from build123d import *

# Parameters (mm, degrees)
F1_DEPTH  = 12.7
F1_FACE_R = 30.3566666554
F2_DEPTH  = 12.7


with BuildPart() as f1:
    # F0 (on Front) → F1 (new body)
    with BuildSketch(Plane.XZ):
        with BuildLine():
            ThreePointArc((-9.3004843115, 36.7589222648), (-23.2923661717, -29.9196098341), (37.9172437619, 0))
            ThreePointArc((37.9172437619, 0), (29.338119554, 24.020660181), (7.4829580234, 37.1715309574))
            Line((7.4829580234, 37.1715309574), (0, 30.3566666554))
            Line((0, 30.3566666554), (-9.3004843115, 36.7589222648))
        make_face()
        with BuildLine():
            ThreePointArc((30.3566666554, 0), (-21.4654048463, -21.4654048463), (0, 30.3566666554))
            ThreePointArc((0, 30.3566666554), (21.4654048463, 21.4654048463), (30.3566666554, 0))
        make_face(mode=Mode.SUBTRACT)
        with BuildLine():
            Line((0, 30.3566666554), (7.4829580234, 37.1715309574))
            ThreePointArc((7.4829580234, 37.1715309574), (-0.9318862244, 37.9057906205), (-9.3004843115, 36.7589222648))
            Line((-9.3004843115, 36.7589222648), (0, 30.3566666554))
        make_face()
        with BuildLine():
            ThreePointArc((-9.3004843115, 36.7589222648), (-0.9318862244, 37.9057906205), (7.4829580234, 37.1715309574))
            Line((7.4829580234, 37.1715309574), (20.2197378858, 48.7711451921))
            ThreePointArc((20.2197378858, 48.7711451921), (11.7747091364, 46.8406854256), (3.6217325155, 49.7688516961))
            ThreePointArc((3.6217325155, 49.7688516961), (-6.3831384952, 42.0012170686), (-18.9701891405, 43.4153414263))
            Line((-18.9701891405, 43.4153414263), (-9.3004843115, 36.7589222648))
        make_face()
        with BuildLine():
            ThreePointArc((3.6217325155, 49.7688516961), (11.7747091364, 46.8406854256), (20.2197378858, 48.7711451921))
            Line((20.2197378858, 48.7711451921), (25.3996234387, 53.4885600209))
            Line((25.3996234387, 53.4885600209), (0, 70.9731206298))
            ThreePointArc((0, 70.9731206298), (4.3420940931, 65.2280612526), (5.8836441513, 58.193637909))
            ThreePointArc((5.8836441513, 58.193637909), (5.3083274131, 53.8320651714), (3.6217325155, 49.7688516961))
        make_face()
        with BuildLine():
            Line((25.3996234387, 53.4885600209), (20.2197378858, 48.7711451921))
            ThreePointArc((20.2197378858, 48.7711451921), (23.0811869033, 50.8317293109), (25.3996234387, 53.4885600209))
        make_face()
        with BuildLine():
            ThreePointArc((-21.873843285, 45.4141551882), (-20.4745226574, 44.3384727889), (-18.9701891405, 43.4153414263))
            Line((-18.9701891405, 43.4153414263), (-21.873843285, 45.4141551882))
        make_face()
        with BuildLine():
            Line((-21.873843285, 45.4141551882), (-18.9701891405, 43.4153414263))
            ThreePointArc((-18.9701891405, 43.4153414263), (-6.3831384952, 42.0012170686), (3.6217325155, 49.7688516961))
            ThreePointArc((3.6217325155, 49.7688516961), (-2.498029855, 59.6350178914), (0, 70.9731206298))
            Line((0, 70.9731206298), (-21.873843285, 45.4141551882))
        make_face()
        with BuildLine():
            Line((0, 70.9731206298), (25.3996234387, 53.4885600209))
            ThreePointArc((25.3996234387, 53.4885600209), (27.4225414081, 57.653295881), (28.1177455183, 62.2308403254))
            ThreePointArc((28.1177455183, 62.2308403254), (17.2773561637, 76.9535700141), (0, 70.9731206298))
        make_face()
        with BuildLine():
            ThreePointArc((0, 70.9731206298), (-2.498029855, 59.6350178914), (3.6217325155, 49.7688516961))
            ThreePointArc((3.6217325155, 49.7688516961), (5.3083274131, 53.8320651714), (5.8836441513, 58.193637909))
            ThreePointArc((5.8836441513, 58.193637909), (4.3420940931, 65.2280612526), (0, 70.9731206298))
        make_face()
        with BuildLine():
            ThreePointArc((0, 70.9731206298), (-23.7164043633, 69.1305595515), (-21.873843285, 45.4141551882))
            Line((-21.873843285, 45.4141551882), (0, 70.9731206298))
        make_face()
    extrude(amount=-F1_DEPTH)

    # F0 (on Front) + F1_face (on face) → F2 (join)
    with BuildSketch(Plane.XZ):
        with BuildLine():
            ThreePointArc((-9.3004843115, 36.7589222648), (-23.2923661717, -29.9196098341), (37.9172437619, 0))
            ThreePointArc((37.9172437619, 0), (29.338119554, 24.020660181), (7.4829580234, 37.1715309574))
            Line((7.4829580234, 37.1715309574), (0, 30.3566666554))
            Line((0, 30.3566666554), (-9.3004843115, 36.7589222648))
        make_face()
        with BuildLine():
            ThreePointArc((30.3566666554, 0), (-21.4654048463, -21.4654048463), (0, 30.3566666554))
            ThreePointArc((0, 30.3566666554), (21.4654048463, 21.4654048463), (30.3566666554, 0))
        make_face(mode=Mode.SUBTRACT)
        with BuildLine():
            Line((0, 30.3566666554), (7.4829580234, 37.1715309574))
            ThreePointArc((7.4829580234, 37.1715309574), (-0.9318862244, 37.9057906205), (-9.3004843115, 36.7589222648))
            Line((-9.3004843115, 36.7589222648), (0, 30.3566666554))
        make_face()
        with BuildLine():
            ThreePointArc((-9.3004843115, 36.7589222648), (-0.9318862244, 37.9057906205), (7.4829580234, 37.1715309574))
            Line((7.4829580234, 37.1715309574), (20.2197378858, 48.7711451921))
            ThreePointArc((20.2197378858, 48.7711451921), (11.7747091364, 46.8406854256), (3.6217325155, 49.7688516961))
            ThreePointArc((3.6217325155, 49.7688516961), (-6.3831384952, 42.0012170686), (-18.9701891405, 43.4153414263))
            Line((-18.9701891405, 43.4153414263), (-9.3004843115, 36.7589222648))
        make_face()
        with BuildLine():
            ThreePointArc((3.6217325155, 49.7688516961), (11.7747091364, 46.8406854256), (20.2197378858, 48.7711451921))
            Line((20.2197378858, 48.7711451921), (25.3996234387, 53.4885600209))
            Line((25.3996234387, 53.4885600209), (0, 70.9731206298))
            ThreePointArc((0, 70.9731206298), (4.3420940931, 65.2280612526), (5.8836441513, 58.193637909))
            ThreePointArc((5.8836441513, 58.193637909), (5.3083274131, 53.8320651714), (3.6217325155, 49.7688516961))
        make_face()
        with BuildLine():
            Line((25.3996234387, 53.4885600209), (20.2197378858, 48.7711451921))
            ThreePointArc((20.2197378858, 48.7711451921), (23.0811869033, 50.8317293109), (25.3996234387, 53.4885600209))
        make_face()
        with BuildLine():
            ThreePointArc((-21.873843285, 45.4141551882), (-20.4745226574, 44.3384727889), (-18.9701891405, 43.4153414263))
            Line((-18.9701891405, 43.4153414263), (-21.873843285, 45.4141551882))
        make_face()
        with BuildLine():
            Line((-21.873843285, 45.4141551882), (-18.9701891405, 43.4153414263))
            ThreePointArc((-18.9701891405, 43.4153414263), (-6.3831384952, 42.0012170686), (3.6217325155, 49.7688516961))
            ThreePointArc((3.6217325155, 49.7688516961), (-2.498029855, 59.6350178914), (0, 70.9731206298))
            Line((0, 70.9731206298), (-21.873843285, 45.4141551882))
        make_face()
        with BuildLine():
            Line((0, 70.9731206298), (25.3996234387, 53.4885600209))
            ThreePointArc((25.3996234387, 53.4885600209), (27.4225414081, 57.653295881), (28.1177455183, 62.2308403254))
            ThreePointArc((28.1177455183, 62.2308403254), (17.2773561637, 76.9535700141), (0, 70.9731206298))
        make_face()
        with BuildLine():
            ThreePointArc((0, 70.9731206298), (-2.498029855, 59.6350178914), (3.6217325155, 49.7688516961))
            ThreePointArc((3.6217325155, 49.7688516961), (5.3083274131, 53.8320651714), (5.8836441513, 58.193637909))
            ThreePointArc((5.8836441513, 58.193637909), (4.3420940931, 65.2280612526), (0, 70.9731206298))
        make_face()
        with BuildLine():
            ThreePointArc((0, 70.9731206298), (-23.7164043633, 69.1305595515), (-21.873843285, 45.4141551882))
            Line((-21.873843285, 45.4141551882), (0, 70.9731206298))
        make_face()
    with BuildSketch(Plane(origin=(0.0200571073, 0, 29.7715951258), x_dir=(1, 0, 0), z_dir=(0, -1, 0))):
        with BuildLine():
            ThreePointArc((20.1996807784, 18.9995500663), (24.0788656265, 42.8406203835), (-0.0200571073, 41.201525504))
            ThreePointArc((-0.0200571073, 41.201525504), (-24.8121438699, 37.9596437982), (-18.9902462478, 13.6437463005))
            Line((-18.9902462478, 13.6437463005), (-9.3205414189, 6.987327139))
            ThreePointArc((-9.3205414189, 6.987327139), (0.9118291171, -67.6773857463), (7.4629009161, 7.3999358316))
            Line((7.4629009161, 7.3999358316), (20.1996807784, 18.9995500663))
        make_face()
        with Locations((-0.0200571073, -29.7715951258)):
            Circle(F1_FACE_R, mode=Mode.SUBTRACT)
    extrude(amount=-F2_DEPTH)


solid = f1.part
Geometry check sheet. Reference: the model listing, model coordinates, mm. Give positions to 0.01 mm unless a question says otherwise; leave off trailing zeros. Order: outer loops, then holes, each group sorted by start corner. A loop starts at its lowest first (then second) coordinate and runs counter-clockwise, first axis right, second up. Notation, with made-up numbers: (27.25, 37.25) - (37.25, 37.25) arc R12 cw to (37.25, 53.25) - close; hole circle Ø5 at (58, -34.5). An arc over 180 degrees is marked (long way). Use one line per item in the form item = value.
1) Sectioned sample at B-B (x = -4). Record the boundary of the cut face in (y, z), and give its area (3 significant figures).
Working result:
outline = (0, -37.71) - (12.7, -37.71) - (12.7, -30.09) - (0, -30.09) - close; (0, 30.09) - (12.7, 30.09) - (12.7, 73.52) - (0, 73.52) - close
area = 648 mm^2
2) Depth check by flat-ended pin: pin 1 Ø8 at (x, z) = (25.5, 14.5) entering from +Y; pin 2 Ø5 at (y, z) = (4, -15) entering from -X; pin 3 Ø10 at (x, z) = (24.5, -4) entering from -Y; pin 4 Ø5 at (y, z) = (9.5, -19) entering from +X. Enter the tip coordinate at first touch or a pass-through.
Working result:
pin_1 = 12.7
pin_2 = -35.8
pin_3 = through
pin_4 = 34.14
3) Draft check along Z on faces 1 (the face through (-1, 0, 34)), 2 (the face through (13.76, 6.26, 42.89)), 3 (the face through (-14.2, 6.26, 40.13)). Enter one of: released by +Z, released by -Z, zero draft, split by the parting line, or undercut.
Working result:
face_1 = zero draft
face_2 = undercut
face_3 = undercut
4) Sectioned sample at D-D (y = 7.5). Record the boundary of the cut face in (x, z), and give its area (3 significant figures).
Working result:
outline = (-18.97, 43.42) - (-9.3, 36.76) arc R37.92 ccw (long way) to (7.48, 37.17) - (20.22, 48.77) arc R15.42 ccw (long way) to (0, 70.97) arc R16.82 ccw (long way) to start; hole circle Ø60.71 at (0, 0)
area = 3,340 mm^2
5) Sectioned sample at C-C (x = 16.5). Record the boundary of the cut face in (y, z).
Working result:
outline = (0, -34.14) - (12.7, -34.14) - (12.7, -25.48) - (0, -25.48) - close; (0, 25.48) - (12.7, 25.48) - (12.7, 34.14) - (0, 34.14) - close; (0, 45.38) - (12.7, 45.38) - (12.7, 77.17) - (0, 77.17) - close
6) Material ranges on probe 1 along Z at (x, y) = (24.5, 3); probe 2 along X at (y, z) = (10.5, 23.5); probe 3 along X at (y, z) = (5.25, -7.5), recorded low to high. Write a range as from..to.
Working result:
probe_1 = -28.94..-17.92, 17.92..28.94, 52.31..72.15
probe_2 = -29.76..-19.22, 19.22..29.76
probe_3 = -37.17..-29.42, 29.42..37.17
7) Sectioned sample at A-A (z = -11). Record the boundary of the cut face in (x, y).
Working result:
outline = (-36.29, 0) - (-28.29, 0) - (-28.29, 12.7) - (-36.29, 12.7) - close; (28.29, 0) - (36.29, 0) - (36.29, 12.7) - (28.29, 12.7) - close
